Check sheet for the modelled part. Datum: model origin and axes. Units: mm. A direction names the side the tool comes from. Round coordinates to 2 decimals unless told otherwise and drop trailing zeros. Write each loop counter-clockwise with the first axis right and the second up, starting at its lowest first coordinate (ties: lowest second). Pieces come first, ordered by that corner, then holes. Notation, with made-up numbers: M 88.25,18.25 L 106.25,18.25 A21 cw 106.25,26.25 Z; hole C -22,-38 d2. An arc over 180 degrees is marked long. Answer in a Markdown table with one row per item.
Solid Edge part; units mm, degrees
sketch "Sketch1" plane through (0, 0, 0) normal (0, -1, 0) x (1, 0, 0)
  line L0 (3.5, 4) -> (3.5, 0)
  line L1 (3.5, 0) -> (2.35, 0)
  line L2 (2.35, 0) -> (2, -0.6062)
  line L3 (2, -0.6062) -> (2, -20)
  line L4 (2, -20) -> (0, -20)
  line L5 (1.5, 2) -> (0, 1.834)
  line L6 (1.5, 4) -> (1.5, 2)
  line L7 (3.5, 4) -> (1.5, 4)
revolve "RevolvedProtrusion1" add sketch "Sketch1" angle 360 about axis through (0, 0, -6) along (0, 0, 1)
cosmetic_thread "Thread1"
chamfer "Chamfer_1" distance 0.4 angle 45 1 edges at (-2, 0, -20)
fillet "Round_1" radius 0.4 2 edges at (-3.5, 0, 0) (-3.5, 0, 4)
sketch "Sketch2" plane through (0, 0, 4) normal (0, 0, 1) x (0, 1, 0)
  line L0 (-1.5, 0.866) -> (-1.5, -0.866)
  line L1 (0, -1.7321) -> (-1.5, -0.866)
  line L2 (1.5, -0.866) -> (0, -1.7321)
  line L3 (1.5, 0.866) -> (1.5, -0.866)
  line L4 (0, 1.7321) -> (1.5, 0.866)
  line L5 (-1.5, 0.866) -> (0, 1.7321)
extrude "Cutout1" cut sketch "Sketch2" against normal up to vertex (2 mm away)
properties material "Galvanized steel"
1. Access from +Z, -Z, +X, -X, +Y, -Y to the whole of each face (thin tool, end or side, straight path). Record for faces 1 (the face through (0, -1.5, 3)), 2 (the face through (0, 0, -20)), 3 (the face through (-2, 2, 0)).
Found:
| item | result |
|---|---|
| face 1 | +Z |
| face 2 | -Z, +X, -X, +Y, -Y |
| face 3 | -Z |
2. Draft check along X on faces 4 (the face through (1.3, -1.3, 4)), 5 (the face through (0, 2, -10)), 6 (the face through (-1.305, 0.74, 3.014)). Enter one of: +X half, -X half, draft (parallel to the pull), parting line (faces both ways), or undercut.
Found:
| item | result |
|---|---|
| face 4 | draft |
| face 5 | parting line |
| face 6 | undercut |
3. Section check A-A, the plane z = -6.75. Record the cut outline in (x, y), and give its area (3 significant figures).
Found:
| item | result |
|---|---|
| outline | C 0,0 d4 |
| area | 12.6 mm2 |
4. Go/stop test with a flat-tipped pin: pin 1 (2 mm diameter, centred on x = -1, z = -2, fed in from +Y). Record where the tip stops, or that it passes through.
Found:
| item | result |
|---|---|
| pin 1 | stops at y = 2 |
5. Scan lines: L1, parallel to Z at x = -2, y = 2; L2, parallel to Z at x = -1.25, y = -0.75; L3, parallel to Y at x = -1, z = -14. Record each from-to range of solid material in increasing order.
Found:
| item | result |
|---|---|
| L1 | z = 0 to 4 |
| L2 | z = -20 to 2 |
| L3 | y = -1.73 to 1.73 |
